Check sheet for the modelled part. Datum: model origin and axes. Units: mm. Round coordinates to 2 decimals unless told otherwise and drop trailing zeros. Write each loop counter-clockwise with the first axis right and the second up, starting at its lowest first coordinate (ties: lowest second). Pieces come first, ordered by that corner, then holes.
Item 1: Cross-section at A-A on z = 1.6. Enter the section's corners in (x, y).
Item 2: Material ranges on line 1 (Y direction, x = -130.5, z = 0.4); line 2 (X direction, y = -5, z = 0.8); line 3 (X direction, y = -2.5, z = 0.7), recorded low to high.
Item 3: Cross-section at B-B on y = 1.5. Enter the section's corners in (x, z).
from build123d import *

# Parameters (mm, degrees)
SKETCH1_W           = 50
SKETCH1_H           = 320
BOSS_EXTRUDE1_DEPTH = 2.4
FILLET1_R           = 10
CHAMFER1_SIZE       = 0.4


with BuildPart() as part:
    # Sketch1 → Boss-Extrude1 (new body)
    with BuildSketch(Plane(origin=(0, 0, 0), x_dir=(0, 1, 0), z_dir=(0, 0, 1))):
        with Locations((2, 0)):
            Rectangle(SKETCH1_W, SKETCH1_H)
        with BuildLine():
            Line((-6, 128.75), (-6, 131.25))
            ThreePointArc((-6, 131.25), (0, 137.25), (6, 131.25))
            Line((6, 131.25), (6, 128.75))
            ThreePointArc((6, 128.75), (0, 122.75), (-6, 128.75))
        make_face(mode=Mode.SUBTRACT)
        with BuildLine():
            Line((-6, -131.25), (-6, -128.75))
            ThreePointArc((-6, -128.75), (0, -122.75), (6, -128.75))
            Line((6, -128.75), (6, -131.25))
            ThreePointArc((6, -131.25), (0, -137.25), (-6, -131.25))
        make_face(mode=Mode.SUBTRACT)
        with BuildLine():
            Line((-2, 1.25), (-2, -1.25))
            ThreePointArc((-2, -1.25), (-7, -6.25), (-12, -1.25))
            Line((-12, -1.25), (-12, 1.25))
            ThreePointArc((-12, 1.25), (-7, 6.25), (-2, 1.25))
        make_face(mode=Mode.SUBTRACT)
    extrude(amount=BOSS_EXTRUDE1_DEPTH)

    # Fillet1
    fillet1_edges = [part.edges().sort_by_distance(p)[0] for p in [
        (160, 27, 1.2),
        (160, -23, 1.2),
        (-160, -23, 1.2),
        (-160, 27, 1.2),
    ]]
    fillet(fillet1_edges, radius=FILLET1_R)

    # Chamfer1
    chamfer1_edges = [part.edges().sort_by_distance(p)[0] for p in [
        (0, 27, 0),
        (0, 27, 2.4),
        (160, 2, 0),
        (0, -23, 0),
        (-160, 2, 0),
        (157.071067812, -20.071067812, 0),
        (-157.071067812, -20.071067812, 0),
        (-157.071067812, 24.071067812, 0),
        (157.071067812, 24.071067812, 0),
        (160, 2, 2.4),
        (-160, 2, 2.4),
        (0, -23, 2.4),
        (157.071067812, -20.071067812, 2.4),
        (-157.071067812, -20.071067812, 2.4),
        (-157.071067812, 24.071067812, 2.4),
        (157.071067812, 24.071067812, 2.4),
    ]]
    chamfer(chamfer1_edges, length=CHAMFER1_SIZE)


solid = part.part
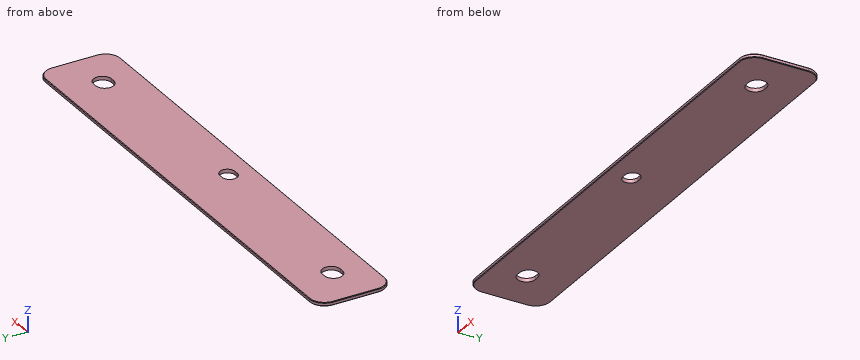
Response values:
1. outline: (-160, -13) arc R10 ccw to (-150, -23) - (150, -23) arc R10 ccw to (160, -13) - (160, 17) arc R10 ccw to (150, 27) - (-150, 27) arc R10 ccw to (-160, 17) - close; hole (-131.25, -6) - (-128.75, -6) arc R6 ccw to (-128.75, 6) - (-131.25, 6) arc R6 ccw to start; hole (-1.25, -12) - (1.25, -12) arc R5 ccw to (1.25, -2) - (-1.25, -2) arc R5 ccw to start; hole (128.75, -6) - (131.25, -6) arc R6 ccw to (131.25, 6) - (128.75, 6) arc R6 ccw to start
2. line 1: y = -23 to -6, 6 to 27
2. line 2: x = -160 to -134.57, -125.43 to -5.83, 5.83 to 125.43, 134.57 to 160
2. line 3: x = -160 to -136.7, -123.3 to -3.43, 3.43 to 123.3, 136.7 to 160
3. outline: (-160, 0.4) - (-159.6, 0) - (-137.06, 0) - (-137.06, 2.4) - (-159.6, 2.4) - (-160, 2) - close; (-122.94, 0) - (122.94, 0) - (122.94, 2.4) - (-122.94, 2.4) - close; (137.06, 0) - (159.6, 0) - (160, 0.4) - (160, 2) - (159.6, 2.4) - (137.06, 2.4) - close
